Geometry check sheet. Reference: the model listing, model coordinates, mm. Face numbers are marked on the shaded views. A direction names the side the tool comes from. Round coordinates to 2 decimals unless told otherwise and drop trailing zeros. Order: outer loops, then holes, each group sorted by start corner. A loop starts at its lowest first (then second) coordinate and runs counter-clockwise, first axis right, second up.
```python
from build123d import *

# Parameters (mm, degrees)
F1_DEPTH = 50.8
F2_W     = 20.32
F2_H     = 38.1
F3_DEPTH = 50.8


with BuildPart() as f1:
    # F0 (on Top) → F1 (new body)
    with BuildSketch(Plane.XY):
        Polygon((0, 0), (-114.3, 0), (-114.3, -12.7), (-101.6, -12.7), (-101.6, -63.5), (-114.3, -63.5), (-114.3, -76.2), (0, -76.2), (0, -63.5), (-12.7, -63.5), (-12.7, -12.7), (0, -12.7), align=None)
    extrude(amount=F1_DEPTH)

    # F2 (on face) → F3 (cut)
    with BuildSketch(Plane.XY.offset(50.8)):
        with Locations((-34.606382, -36.83)):
            Rectangle(F2_W, F2_H)
        with Locations((-55.689771, -36.83)):
            Rectangle(F2_W, F2_H)
        with Locations((-79.693612, -36.83)):
            Rectangle(F2_W, F2_H)
    extrude(amount=-F3_DEPTH, mode=Mode.SUBTRACT)


solid = f1.part
```
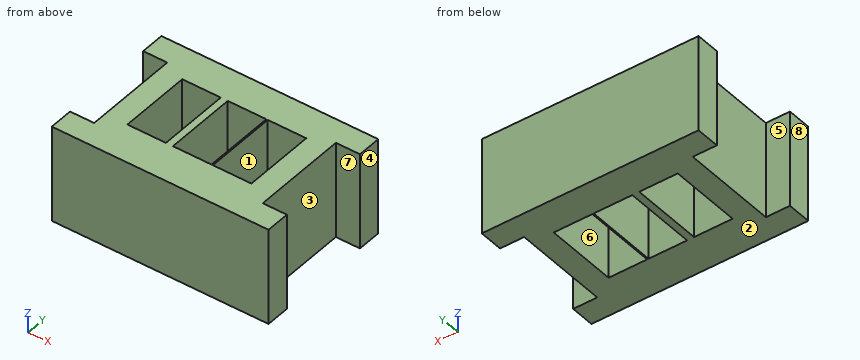
(1) Set-up check for the marked faces 4, 5, 6, 7 and 8: record each of +Z, -Z, +X, -X, +Y, -Y from which the full face is reachable in a straight line by a thin tool's end or side.
Returned:
face 4: +Z, -Z, +X, +Y, -Y
face 5: +Z, -Z, -X
face 6: +Z, -Z
face 7: +Z, -Z, +X
face 8: +Z, -Z, -X, +Y, -Y
(2) Material ranges on line 1 (X direction, y = -46.5, z = 18); line 2 (Y direction, x = -28, z = 10); line 3 (X direction, y = -61, z = 8), recorded low to high.
Returned:
line 1: x = -101.6 to -89.85, -69.53 to -65.85, -45.53 to -44.77, -24.45 to -12.7
line 2: y = -76.2 to -55.88, -17.78 to 0
line 3: x = -101.6 to -12.7
(3) Sectioned sample at A-A, the plane x = -75. Record the cut outline in (y, z).
Returned:
outline: (-76.2, 0) - (-55.88, 0) - (-55.88, 50.8) - (-76.2, 50.8) - close; (-17.78, 0) - (0, 0) - (0, 50.8) - (-17.78, 50.8) - close
(4) Draft check along X on the marked faces 1, 2 and 3. Enter one of: released by +X, released by -X, zero draft, split by the parting line, or undercut.
Returned:
face 1: undercut
face 2: zero draft
face 3: released by +X
(5) Sectioned sample at B-B, the plane z = 16. Record the cut outline in (x, y).
Returned:
outline: (-114.3, -76.2) - (0, -76.2) - (0, -63.5) - (-12.7, -63.5) - (-12.7, -12.7) - (0, -12.7) - (0, 0) - (-114.3, 0) - (-114.3, -12.7) - (-101.6, -12.7) - (-101.6, -63.5) - (-114.3, -63.5) - close; hole (-89.85, -55.88) - (-69.53, -55.88) - (-69.53, -17.78) - (-89.85, -17.78) - close; hole (-65.85, -55.88) - (-45.53, -55.88) - (-45.53, -17.78) - (-65.85, -17.78) - close; hole (-44.77, -55.88) - (-24.45, -55.88) - (-24.45, -17.78) - (-44.77, -17.78) - close
(6) Sectioned sample at C-C, the plane y = -39. Record the cut outline in (x, z), and give its area (3 significant figures).
Returned:
outline: (-101.6, 0) - (-89.85, 0) - (-89.85, 50.8) - (-101.6, 50.8) - close; (-69.53, 0) - (-65.85, 0) - (-65.85, 50.8) - (-69.53, 50.8) - close; (-45.53, 0) - (-44.77, 0) - (-44.77, 50.8) - (-45.53, 50.8) - close; (-24.45, 0) - (-12.7, 0) - (-12.7, 50.8) - (-24.45, 50.8) - close
area: 1,420 mm2
(7) Depth check by flat-ended pin: P1, Ø2, axis at y = -12.5, z = 27.5, coming from the +X side; P2, Ø8, axis at y = -28, z = 44.5, coming from the +X side; P3, Ø4, axis at y = -36, z = 24, coming from the -X side. Enter the tip coordinate at first touch or a pass-through.
Returned:
P1: stops at x = 0
P2: stops at x = -12.7
P3: stops at x = -101.6
(8) Sectioned sample at D-D, the plane x = -10. Record the cut outline in (y, z).
Returned:
outline: (-76.2, 0) - (-63.5, 0) - (-63.5, 50.8) - (-76.2, 50.8) - close; (-12.7, 0) - (0, 0) - (0, 50.8) - (-12.7, 50.8) - close
